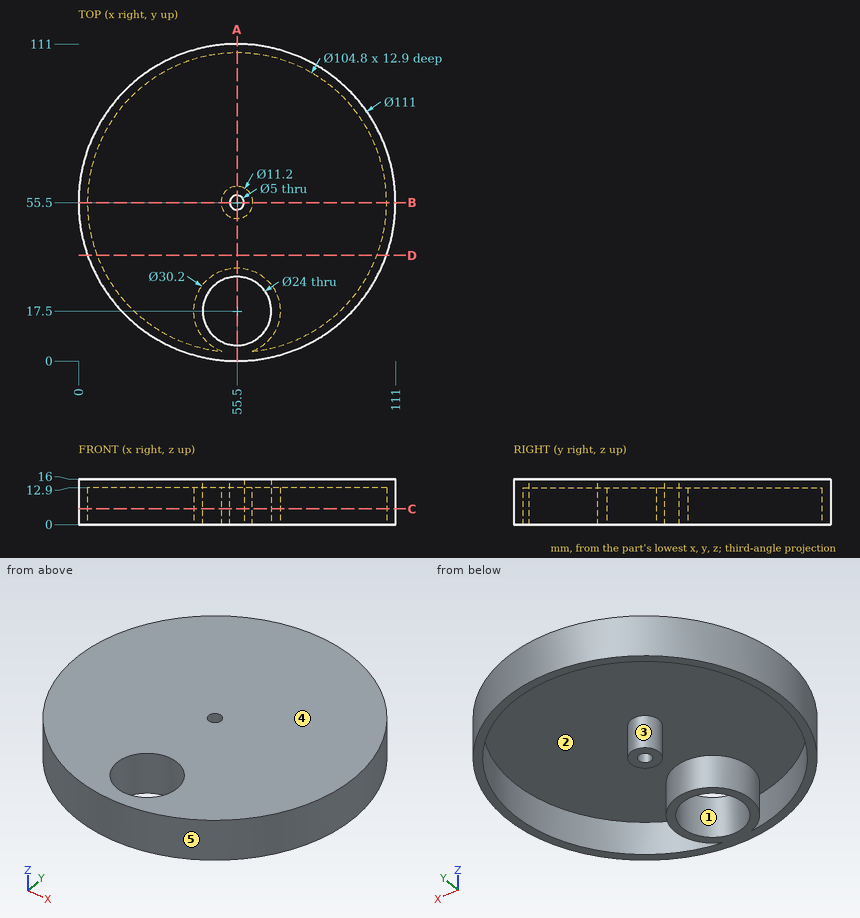
Geometry check sheet. Reference: drawing and pictorial views, mm from the part's lowest x, y, z. A direction names the side the tool comes from. Give positions to 0.01 mm unless a question says otherwise; leave off trailing zeros. Write each loop counter-clockwise with the first axis right and the second up, starting at its lowest first coordinate (ties: lowest second). Pieces come first, ordered by that corner, then holes. Notation, with made-up numbers: (26.25, 60.5) - (84.25, 60.5) arc R30 cw to (84.25, 83.5) - close; hole circle Ø9 at (68.25, 40.5). An arc over 180 degrees is marked (long way). Put each result on its own line as item: value.
Q1. Section check A-A on x = 55.5. Record the cut outline in (y, z).
Result:
outline: (0, 0) - (5.5, 0) - (5.5, 16) - (0, 16) - close; (29.5, 0) - (32.6, 0) - (32.6, 12.9) - (49.9, 12.9) - (49.9, 0) - (53, 0) - (53, 16) - (29.5, 16) - close; (58, 0) - (61.1, 0) - (61.1, 12.9) - (107.9, 12.9) - (107.9, 0) - (111, 0) - (111, 16) - (58, 16) - close
Q2. Scan lines: probe 1 along Y at (x, z) = (55.5, 12.25); probe 2 along Y at (x, z) = (52, 2.5); probe 3 along X at (y, z) = (26, 5.5). Record each from-to range of solid material in increasing order. Write a range as from..to.
Result:
probe 1: 0..5.5, 29.5..32.6, 49.9..53, 58..61.1, 107.9..111
probe 2: 0.11..6.02, 28.98..32.19, 51.13..59.87, 107.78..110.89
probe 3: 8.49..12.19, 43.02..47.03, 63.97..67.98, 98.81..102.51
Q3. Mould release check, pull along Y, two halves, no side actions. Record for the marked faces 3, 4 and 5: released by +Y, released by -Y, zero draft, split by the parting line, or undercut.
Result:
face 3: undercut
face 4: zero draft
face 5: split by the parting line
Q4. Set-up check for the marked faces 1 and 2: record each of +Z, -Z, +X, -X, +Y, -Y from which the full face is reachable in a straight line by a thin tool's end or side.
Result:
face 1: +Z, -Z
face 2: -Z
Q5. Section check D-D on y = 37. Record the cut outline in (x, z).
Result:
outline: (3.17, 0) - (6.47, 0) - (6.47, 12.9) - (104.53, 12.9) - (104.53, 0) - (107.83, 0) - (107.83, 16) - (3.17, 16) - close
Q6. Depth check by flat-ended pin: P1, Ø8, axis at x = 89, y = 43, coming from the -Z side; P2, Ø6, axis at y = 12, z = 10.5, coming from the -X side; P3, Ø6, axis at x = 48.5, z = 2, coming from the +Y side. Enter the tip coordinate at first touch or a pass-through.
Result:
P1: z = 12.9
P2: x = 17.55
P3: y = 110.86
Q7. Section check C-C on z = 5.5. Record the cut outline in (x, y).
Result:
outline: circle Ø111 at (55.5, 55.5); circle Ø11.2 at (55.5, 55.5); hole circle Ø24 at (55.5, 17.5); hole (50.17, 3.37) arc R15.1 cw (long way) to (60.83, 3.37) arc R52.4 ccw (long way) to start; hole circle Ø5 at (55.5, 55.5)
Q8. Section check B-B on y = 55.5. Record the cut outline in (x, z).
Result:
outline: (0, 0) - (3.1, 0) - (3.1, 12.9) - (49.9, 12.9) - (49.9, 0) - (53, 0) - (53, 16) - (0, 16) - close; (58, 0) - (61.1, 0) - (61.1, 12.9) - (107.9, 12.9) - (107.9, 0) - (111, 0) - (111, 16) - (58, 16) - close
